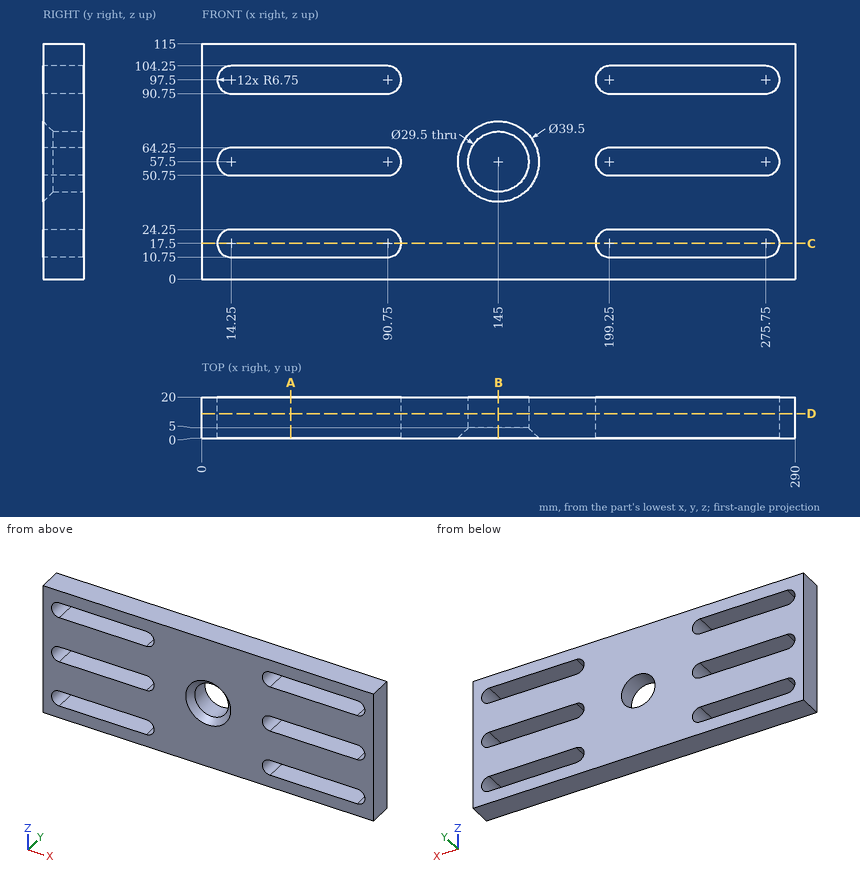
Check sheet for the drawn part. Datum: minimum x, y, z corner. Units: mm. Round coordinates to 2 decimals unless told otherwise and drop trailing zeros. Loops run counter-clockwise (first coordinate to the right, second up) from the corner with the lowest first, then second, coordinate; pieces in that order, holes last. Notation, with made-up numbers: (79, 20) - (111, 20) arc R10 ccw to (111, 38) - close; hole circle Ø9 at (11.5, 83). An arc over 180 degrees is marked (long way). Write item = value, one per line. Start each with the question number.
1. Depth check by flat-ended pin: pin 1 (1 mm diameter, centred on x = 254, z = 32.5, fed in from -Y). Enter the tip coordinate at first touch or a pass-through.
2. Section check C-C on z = 17.5. Enter the section's corners in (x, y), then the cut area to 3 significant figures.
3. Section check D-D on y = 12. Give the number of separate pieces and of enclosed holes in the cut face, then the cut area to 3 significant figures.
4. Section check A-A on x = 43.5. Enter the section's corners in (y, z).
5. Thickness scan on line 1 (Z direction, x = 19.5, y = 17); line 2 (X direction, y = 14.75, z = 57.5); line 3 (Z direction, x = 96, y = 8). Record the ranges inside material, lowest first.
6. Section check B-B on x = 145. Enter the section's corners in (y, z), then the cut area to 4 significant figures.
Working result:
q1.pin_1 = 0
q2.outline = (0, 0) - (7.5, 0) - (7.5, 20) - (0, 20) - close; (97.5, 0) - (192.5, 0) - (192.5, 20) - (97.5, 20) - close; (282.5, 0) - (290, 0) - (290, 20) - (282.5, 20) - close
q2.area = 2,200 mm^2
q3.separate_pieces = 1
q3.enclosed_holes = 7
q3.area = 25,600 mm^2
q4.outline = (0, 0) - (20, 0) - (20, 10.75) - (0, 10.75) - close; (0, 24.25) - (20, 24.25) - (20, 50.75) - (0, 50.75) - close; (0, 64.25) - (20, 64.25) - (20, 90.75) - (0, 90.75) - close; (0, 104.25) - (20, 104.25) - (20, 115) - (0, 115) - close
q5.line_1 = 0 to 10.75, 24.25 to 50.75, 64.25 to 90.75, 104.25 to 115
q5.line_2 = 0 to 7.5, 97.5 to 130.25, 159.75 to 192.5, 282.5 to 290
q5.line_3 = 0 to 13.26, 21.74 to 53.26, 61.74 to 93.26, 101.74 to 115
q6.outline = (0, 0) - (20, 0) - (20, 42.75) - (5, 42.75) - (0, 37.75) - close; (0, 77.25) - (5, 72.25) - (20, 72.25) - (20, 115) - (0, 115) - close
q6.area = 1,685 mm^2
